Design review of the part built by this model. Coordinates are the model's own, in mm. A direction names the side the tool comes from. Give positions to 0.01 mm unless a question says otherwise; leave off trailing zeros. Write each loop counter-clockwise with the first axis right and the second up, starting at its lowest first coordinate (ties: lowest second). Pieces come first, ordered by that corner, then holes. Notation, with made-up numbers: (10, -14) -> (60, -14) arc R22 cw to (60, -4) -> close; hole circle Ø8 at (65, -18). An arc over 180 degrees is marked (long way). Answer as a JSON object with one key per item and string values.
```python
from build123d import *

# Parameters (mm, degrees)
SKETCH1_W           = 60
SKETCH1_H           = 30
SKETCH1_R           = 12.5
BOSS_EXTRUDE2_DEPTH = 20
SKETCH2_R           = 4
CUT_EXTRUDE1_DEPTH  = 10


with BuildPart() as part:
    # Sketch1 → Boss-Extrude2 (new body)
    with BuildSketch(Plane.XY):
        with Locations((2.571428571, 3)):
            Rectangle(SKETCH1_W, SKETCH1_H)
        with Locations((2.571428571, 3)):
            Circle(SKETCH1_R, mode=Mode.SUBTRACT)
    extrude(amount=BOSS_EXTRUDE2_DEPTH)

    # Sketch2 → Cut-Extrude1 (cut)
    with BuildSketch(Plane.XZ.offset(12)):
        with Locations((-20.428571429, 10)):
            Circle(SKETCH2_R)
        with Locations((25.571428571, 10)):
            Circle(SKETCH2_R)
    extrude(amount=-CUT_EXTRUDE1_DEPTH, mode=Mode.SUBTRACT)


solid = part.part
```
(1) For faces 1 (the cylindrical face through (21.575, -7.07, 10.176)), 2 (the flat face through (-11, 3, 20)), list the 3-axis set-ups (+Z, -Z, +X, -X, +Y, -Y) from which the entire face can be reached by the end or side of a thin tool; tool diameter is ignored.
Here are the results:
{"face 1": "-Y", "face 2": "+Z, +X, -X, +Y, -Y"}
(2) We need section B-B, the plane z = 16. State the section outline as (x, y) points, then the cut area to 3 significant figures.
Here are the results:
{"outline": "(-27.43, -12) -> (32.57, -12) -> (32.57, 18) -> (-27.43, 18) -> close; hole circle Ø25 at (2.57, 3)", "area": "1,310 mm²"}
(3) We need section A-A, the plane y = 3. State the section outline as (x, z) points.
Here are the results:
{"outline": "(-27.43, 0) -> (-9.93, 0) -> (-9.93, 20) -> (-27.43, 20) -> close; (15.07, 0) -> (32.57, 0) -> (32.57, 20) -> (15.07, 20) -> close"}
(4) For line 1 along X through (y, z) = (-5.25, 9.25); line 2 along Y through (x, z) = (5.5, 14); line 3 along X through (y, z) = (-6.75, 15), list the stretches that pass through material, from the lowest coordinate up.
Here are the results:
{"line 1": "x = -27.43 to -24.36, -16.5 to -6.82, 11.96 to 21.64, 29.5 to 32.57", "line 2": "y = -12 to -9.15, 15.15 to 18", "line 3": "x = -27.43 to -5.25, 10.39 to 32.57"}
(5) The part is to be moulded in two halves that separate along X. For faces 3 (the flat face through (26, -2, 10)), 4 (the flat face through (-27.429, 3, 10)), 5 (the flat face through (-20, -2, 10)), 6 (the flat face through (-11, 3, 0)), say which applies: +X half, -X half, draft (parallel to the pull), parting line (faces both ways), or undercut.
Here are the results:
{"face 3": "undercut", "face 4": "-X half", "face 5": "undercut", "face 6": "draft"}
(6) We need section C-C, the plane y = -6. State the section outline as (x, z) points.
Here are the results:
{"outline": "(-27.43, 0) -> (-6.1, 0) -> (-6.1, 20) -> (-27.43, 20) -> close; (11.25, 0) -> (32.57, 0) -> (32.57, 20) -> (11.25, 20) -> close; hole circle Ø8 at (-20.43, 10); hole circle Ø8 at (25.57, 10)"}
(7) Clearance check with a flat-ended pin moving along its axis: pin 1 (4 mm diameter, centred on x = 24.5, z = 9, fed in from -Y). State where the tip first meets the part, or that it passes through.
Here are the results:
{"pin 1": "stops at y = -2"}
(8) We need section D-D, the plane x = 24.5. State the section outline as (y, z) points, then the cut area to 3 significant figures.
Here are the results:
{"outline": "(-12, 0) -> (18, 0) -> (18, 20) -> (-12, 20) -> (-12, 13.85) -> (-2, 13.85) -> (-2, 6.15) -> (-12, 6.15) -> close", "area": "523 mm²"}
